Could you check a few things on this model? Use its own coordinates, in mm. A direction names the side the tool comes from. Round coordinates to 2 decimals unless told otherwise and drop trailing zeros. Write each loop counter-clockwise with the first axis right and the second up, starting at its lowest first coordinate (ties: lowest second). Pieces come first, ordered by that corner, then holes. Notation, with made-up numbers: (56.5, 27) -> (113.5, 27) arc R33 cw to (113.5, 63) -> close; hole circle Ø5 at (45, 80). An arc over 180 degrees is marked (long way). Answer as CSV lines item,"result". Start each with the question number.
Q1. For faces 1 (the cylindrical face through (175.33, 26.01, 78.88)), 2 (the flat face through (210, 85, 79)), 3 (the flat face through (-10, 85, 79)), which set-ups out of +Z, -Z, +X, -X, +Y, -Y let a thin tool reach every point of the face, with its end or its side?
Q2. If I drill on line 1 (Y direction, x = 105, z = 55.5); line 2 (X direction, y = 59, z = 39.5); line 3 (X direction, y = 32, z = 74), over which ranges is the centre line in solid material (lowest first)? Write a range as [from, to].
Q3. Imagine slicing it at D-D on y = 69.5. Please give me the cut outline in (x, z), and give its area (3 significant figures).
Q4. Imagine slicing it at A-A on z = 20. Please give me the cut outline in (x, y).
Q5. Will these pins go through, and if not, where does the flat tip stop? pin 1 Ø2 at (y, z) = (57.5, 137.5) entering from -X; pin 2 Ø8 at (x, z) = (-10, 112.5) entering from -Y; pin 3 Ø5 at (y, z) = (19.5, 140.5) entering from -X.
Q6. Imagine slicing it at B-B on y = 45.5. Please give me the cut outline in (x, z), and give its area (3 significant figures).
Q7. Imagine slicing it at C-C on z = 148.5. Please give me the cut outline in (x, y).
Q8. If we mould it in two halves opening along Z, with no side actions, what happens to faces 4 (the flat face through (99, -3, 0)), 5 (the flat face through (-7, 90, 79)), 6 (the cylindrical face through (207.615, 87.465, 20.105))? For each: pulls with the +Z half, pulls with the -Z half, needs draft (parallel to the pull), parting line crosses it, or undercut.
from build123d import *

# Parameters (mm, degrees)
BOSS_EXTRUDE1_DEPTH = 160
SKETCH2_R           = 2.38125
CUT_EXTRUDE1_DEPTH  = 160


with BuildPart() as part:
    # Sketch1 → Boss-Extrude1 (new body)
    with BuildSketch(Plane.XY):
        with BuildLine():
            Line((113.5, 0), (86.5, 0))
            ThreePointArc((86.5, 0), (25.335263427, 25.335263427), (0, 86.5))
            Line((0, 86.5), (0, 90))
            Line((0, 90), (-15, 90))
            Line((-15, 90), (-15, 85))
            Line((-15, 85), (-4.987704092, 85))
            ThreePointArc((-4.987704092, 85), (22.332251091, 21.271555285), (86.5, -5))
            Line((86.5, -5), (113.5, -5))
            ThreePointArc((113.5, -5), (177.667748909, 21.271555285), (204.987704092, 85))
            Line((204.987704092, 85), (215, 85))
            Line((215, 85), (215, 90))
            Line((215, 90), (200, 90))
            Line((200, 90), (200, 86.5))
            ThreePointArc((200, 86.5), (174.664736573, 25.335263427), (113.5, 0))
        make_face()
    extrude(amount=BOSS_EXTRUDE1_DEPTH)

    # Sketch2 → Cut-Extrude1 (cut)
    with BuildSketch(Plane.XZ.offset(-85)):
        with BuildLine():
            ThreePointArc((-9.993852046, 142.38125), (-12.375102046, 140), (-9.993852046, 137.61875))
            Line((-9.993852046, 137.61875), (-9.993852046, 142.38125))
        make_face()
        with BuildLine():
            Line((-9.993852046, 142.38125), (-9.993852046, 137.61875))
            ThreePointArc((-9.993852046, 137.61875), (-8.310054023, 138.316201977), (-7.612602046, 140))
            ThreePointArc((-7.612602046, 140), (-8.310054023, 141.683798023), (-9.993852046, 142.38125))
        make_face()
        with Locations((-9.993852046, 20)):
            Circle(SKETCH2_R)
        with Locations((209.993852046, 20)):
            Circle(SKETCH2_R)
        with Locations((209.993852046, 140)):
            Circle(SKETCH2_R)
    extrude(amount=-CUT_EXTRUDE1_DEPTH, mode=Mode.SUBTRACT)


solid = part.part
Checks:
1,face 1,"+Z, -Z, +Y"
1,face 2,"+Z, -Z, +X, -Y"
1,face 3,"+Z, -Z, -X, -Y"
2,line 1,"[-5, 0]"
2,line 2,"[-0.77, 4.49], [195.51, 200.77]"
2,line 3,"[13, 19.33], [180.67, 187]"
3,outline,"(-3.41, 0) -> (1.69, 0) -> (1.69, 160) -> (-3.41, 160) -> close; (198.31, 0) -> (203.41, 0) -> (203.41, 160) -> (198.31, 160) -> close"
3,area,"1,630 mm^2"
4,outline,"(-15, 85) -> (-12.38, 85) -> (-12.38, 90) -> (-15, 90) -> close; (-7.61, 85) -> (-4.99, 85) arc R91.5 ccw to (86.5, -5) -> (113.5, -5) arc R91.5 ccw to (204.99, 85) -> (207.61, 85) -> (207.61, 90) -> (200, 90) -> (200, 86.5) arc R86.5 cw to (113.5, 0) -> (86.5, 0) arc R86.5 cw to (0, 86.5) -> (0, 90) -> (-7.61, 90) -> close; (212.38, 85) -> (215, 85) -> (215, 90) -> (212.38, 90) -> close"
5,pin 1,"x = -0.61"
5,pin 2,"y = 85"
5,pin 3,"x = 21.6"
6,outline,"(4.7, 0) -> (10.33, 0) -> (10.33, 160) -> (4.7, 160) -> close; (189.67, 0) -> (195.3, 0) -> (195.3, 160) -> (189.67, 160) -> close"
6,area,"1,800 mm^2"
7,outline,"(-15, 85) -> (-4.99, 85) arc R91.5 ccw to (86.5, -5) -> (113.5, -5) arc R91.5 ccw to (204.99, 85) -> (215, 85) -> (215, 90) -> (200, 90) -> (200, 86.5) arc R86.5 cw to (113.5, 0) -> (86.5, 0) arc R86.5 cw to (0, 86.5) -> (0, 90) -> (-15, 90) -> close"
8,face 4,"pulls with the -Z half"
8,face 5,"needs draft"
8,face 6,"undercut"
